Could you check a few things on this drawing? It's one solid part, dimensions in mm from its lowest x, y, z. A direction names the side the tool comes from. Round coordinates to 2 decimals unless told otherwise and drop trailing zeros. Loops run counter-clockwise (first coordinate to the right, second up) from the corner with the lowest first, then second, coordinate; pieces in that order, holes last.
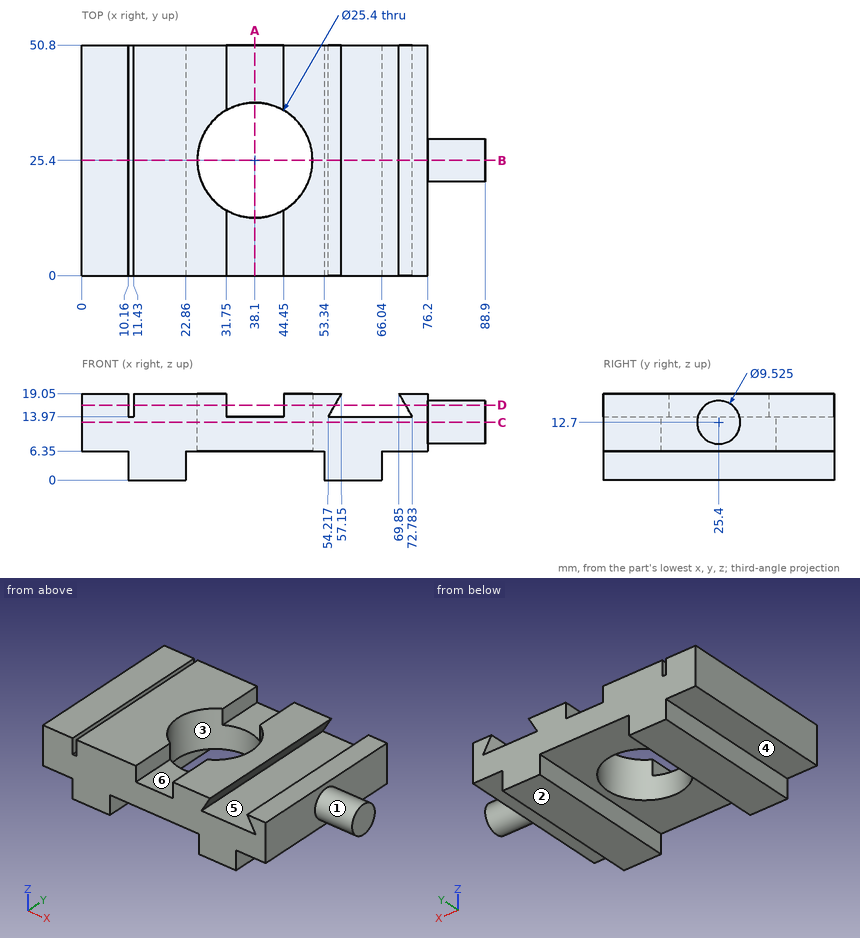
(1) Suppose I cut it at B-B (y = 25.4). Write out the boundary of the cut face in (x, z), then the cut area to 3 significant figures.
(2) Suppose I cut it at C-C (z = 12.7). Write out the boundary of the cut face in (x, y).
(3) Suppose I cut it at A-A (x = 38.1). Write out the boundary of the cut face in (y, z).
(4) Which directions (+Z, -Z, +X, -X, +Y, -Y) give clear straight access to the entire face, cutting with the end or side of a thin tool? Please do the marked faces 4, 5 and 6.
(5) For pin 1 (10 mm diameter, centred on x = 39, y = 9.5, fed in from +Z); pin 2 (5 mm diameter, centred on y = 13, z = 2, fed in from +X); pin 3 (2 mm diameter, centred on y = 15.5, z = 7, fed in from +X), each with a flat end and sliding along its axis, tell me the tip position at first contact or that it passes through.
(6) We'd pull the mould along Y, two halves only. Please class the marked faces 1, 2 and 3: released by +Y, released by -Y, zero draft, split by the parting line, or undercut.
(7) If I drill on line 1 (Y direction, x = 38.1, z = 12); line 2 (X direction, y = 19.5, z = 6.25); line 3 (X direction, y = 25.4, z = 13), over which ranges is the centre line in solid material (lowest first)?
(8) Suppose I cut it at D-D (z = 16.5). Write out the boundary of the cut face in (x, y).
Check result:
1. outline: (0, 6.35) - (10.16, 6.35) - (10.16, 0) - (22.86, 0) - (22.86, 6.35) - (25.4, 6.35) - (25.4, 19.05) - (11.43, 19.05) - (11.43, 13.97) - (10.16, 13.97) - (10.16, 19.05) - (0, 19.05) - close; (50.8, 6.35) - (53.34, 6.35) - (53.34, 0) - (66.04, 0) - (66.04, 6.35) - (76.2, 6.35) - (76.2, 7.94) - (88.9, 7.94) - (88.9, 17.46) - (76.2, 17.46) - (76.2, 19.05) - (69.85, 19.05) - (72.78, 13.97) - (54.22, 13.97) - (57.15, 19.05) - (50.8, 19.05) - close
1. area: 842 mm2
2. outline: (0, 0) - (76.2, 0) - (76.2, 20.64) - (88.9, 20.64) - (88.9, 30.16) - (76.2, 30.16) - (76.2, 50.8) - (0, 50.8) - close; hole circle Ø25.4 at (38.1, 25.4)
3. outline: (0, 6.35) - (12.7, 6.35) - (12.7, 13.97) - (0, 13.97) - close; (38.1, 6.35) - (50.8, 6.35) - (50.8, 13.97) - (38.1, 13.97) - close
4. face 4: -Z, -X, +Y, -Y
4. face 5: +Y, -Y
4. face 6: +Z, +Y, -Y
5. pin 1: stops at z = 13.97
5. pin 2: stops at x = 66.04
5. pin 3: stops at x = 76.2
6. face 1: split by the parting line
6. face 2: zero draft
6. face 3: undercut
7. line 1: y = 0 to 12.7, 38.1 to 50.8
7. line 2: x = 10.16 to 22.86, 53.34 to 66.04
7. line 3: x = 0 to 25.4, 50.8 to 88.9
8. outline: (0, 0) - (10.16, 0) - (10.16, 50.8) - (0, 50.8) - close; (11.43, 0) - (31.75, 0) - (31.75, 14.4) arc R12.7 cw to (31.75, 36.4) - (31.75, 50.8) - (11.43, 50.8) - close; (44.45, 0) - (55.68, 0) - (55.68, 50.8) - (44.45, 50.8) - (44.45, 36.4) arc R12.7 cw to (44.45, 14.4) - close; (71.32, 0) - (76.2, 0) - (76.2, 22.53) - (88.9, 22.53) - (88.9, 28.27) - (76.2, 28.27) - (76.2, 50.8) - (71.32, 50.8) - close
